Geometry: final body of the model. Coordinates: model frame, mm. Face numbers are marked on the shaded views. A direction names the side the tool comes from. Coordinates: 2 decimals unless noted, no trailing zeros. Order: outer loops, then holes, each group sorted by start corner. A loop starts at its lowest first (then second) coordinate and runs counter-clockwise, first axis right, second up. Notation, with made-up numbers: (79, -2) -> (127, -2) arc R19 ccw to (127, 18) -> close; hole circle Ø6 at (65, 46). An arc over 180 degrees is marked (long way). Use CSV: the item, a comma, the result in double quotes. Start each with the question number.
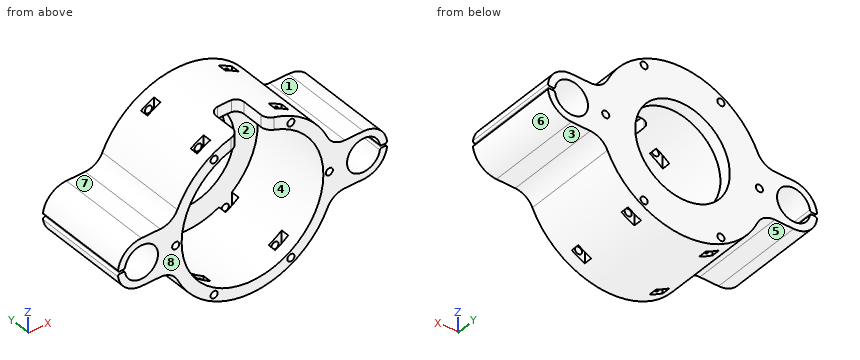
from build123d import *

# Parameters (mm, degrees)
F0_R           = 30
F1_DEPTH       = 35
F0_R_2         = 20
F2_DEPTH       = 5
F5_D           = 3
F4_W           = 12
F4_H           = 10.6380879879
F6_DEPTH       = 15
F7_R           = 3
F8_R           = 0.7
F9_R           = 0.8
F10_W          = 5.5
F10_H          = 3.5
F11_DEPTH      = 50
F11_DEPTH_BACK = 50


with BuildPart() as f1:
    # F0 (on Front) → F1 (new body)
    with BuildSketch(Plane.XZ):
        with BuildLine():
            ThreePointArc((-42.3231782953, 0.5), (-28.3410582734, 0), (-42.3231782953, -0.5))
            Line((-42.3231782953, -0.5), (-45.3285504511, -0.5))
            ThreePointArc((-45.3285504511, -0.5), (-42.2330826494, -7.2456883731), (-35.3410582734, -10))
            Line((-35.3410582734, -10), (-27.3923066529, -10))
            ThreePointArc((-27.3923066529, -10), (-23.0789957248, -11.2623929443), (-20.1269581172, -14.6511627907))
            ThreePointArc((-20.1269581172, -14.6511627907), (11.6589417266, -35), (43.4448415704, -14.6511627907))
            ThreePointArc((43.4448415704, -14.6511627907), (46.396879178, -11.2623929443), (50.7101901061, -10))
            Line((50.7101901061, -10), (58.6589417266, -10))
            ThreePointArc((58.6589417266, -10), (65.5509661026, -7.2456883731), (68.6464339043, -0.5))
            Line((68.6464339043, -0.5), (65.6410617485, -0.5))
            ThreePointArc((65.6410617485, -0.5), (51.6589417266, 0), (65.6410617485, 0.5))
            Line((65.6410617485, 0.5), (68.6464339043, 0.5))
            ThreePointArc((68.6464339043, 0.5), (65.5509661026, 7.2456883731), (58.6589417266, 10))
            Line((58.6589417266, 10), (50.7101901061, 10))
            ThreePointArc((50.7101901061, 10), (46.396879178, 11.2623929443), (43.4448415704, 14.6511627907))
            ThreePointArc((43.4448415704, 14.6511627907), (11.6589417266, 35), (-20.1269581172, 14.6511627907))
            ThreePointArc((-20.1269581172, 14.6511627907), (-23.0789957248, 11.2623929443), (-27.3923066529, 10))
            Line((-27.3923066529, 10), (-35.3410582734, 10))
            ThreePointArc((-35.3410582734, 10), (-42.2330826494, 7.2456883731), (-45.3285504511, 0.5))
            Line((-45.3285504511, 0.5), (-42.3231782953, 0.5))
        make_face()
        with Locations((11.6589417266, 0)):
            Circle(F0_R, mode=Mode.SUBTRACT)
    extrude(amount=F1_DEPTH)

    # F0 (on Front) → F2 (join)
    with BuildSketch(Plane.XZ):
        with BuildLine():
            ThreePointArc((-42.3231782953, 0.5), (-28.3410582734, 0), (-42.3231782953, -0.5))
            Line((-42.3231782953, -0.5), (-45.3285504511, -0.5))
            ThreePointArc((-45.3285504511, -0.5), (-42.2330826494, -7.2456883731), (-35.3410582734, -10))
            Line((-35.3410582734, -10), (-27.3923066529, -10))
            ThreePointArc((-27.3923066529, -10), (-23.0789957248, -11.2623929443), (-20.1269581172, -14.6511627907))
            ThreePointArc((-20.1269581172, -14.6511627907), (11.6589417266, -35), (43.4448415704, -14.6511627907))
            ThreePointArc((43.4448415704, -14.6511627907), (46.396879178, -11.2623929443), (50.7101901061, -10))
            Line((50.7101901061, -10), (58.6589417266, -10))
            ThreePointArc((58.6589417266, -10), (65.5509661026, -7.2456883731), (68.6464339043, -0.5))
            Line((68.6464339043, -0.5), (65.6410617485, -0.5))
            ThreePointArc((65.6410617485, -0.5), (51.6589417266, 0), (65.6410617485, 0.5))
            Line((65.6410617485, 0.5), (68.6464339043, 0.5))
            ThreePointArc((68.6464339043, 0.5), (65.5509661026, 7.2456883731), (58.6589417266, 10))
            Line((58.6589417266, 10), (50.7101901061, 10))
            ThreePointArc((50.7101901061, 10), (46.396879178, 11.2623929443), (43.4448415704, 14.6511627907))
            ThreePointArc((43.4448415704, 14.6511627907), (11.6589417266, 35), (-20.1269581172, 14.6511627907))
            ThreePointArc((-20.1269581172, 14.6511627907), (-23.0789957248, 11.2623929443), (-27.3923066529, 10))
            Line((-27.3923066529, 10), (-35.3410582734, 10))
            ThreePointArc((-35.3410582734, 10), (-42.2330826494, 7.2456883731), (-45.3285504511, 0.5))
            Line((-45.3285504511, 0.5), (-42.3231782953, 0.5))
        make_face()
        with Locations((11.6589417266, 0)):
            Circle(F0_R, mode=Mode.SUBTRACT)
        with Locations((11.6589417266, 0)):
            Circle(F0_R)
        with Locations((11.6589417266, 0)):
            Circle(F0_R_2, mode=Mode.SUBTRACT)
    extrude(amount=-F2_DEPTH)

    # F5 (through all)
    with Locations(Plane.XZ.offset(35)):
        with Locations((-4.5905371539, 28.1467282284), (27.910505085, 28.1467282284), (44.1610262045, 0), (27.910505085, -28.1467282284), (-4.5905371539, -28.1467282284), (-20.8410582734, 0)):
            Hole(F5_D / 2)

    # F4 (on offset) → F6 (cut)
    with BuildSketch(Plane.XZ.offset(35)):
        with Locations((11.6610262045, 32.1714654565)):
            Rectangle(F4_W, F4_H)
    extrude(amount=-F6_DEPTH, mode=Mode.SUBTRACT)

    # F7
    f7_edges = [f1.edges().sort_by_distance(p)[0] for p in [
        (5.661026, -20, 31.938272),
        (17.661026, -20, 31.937484),
        (5.661026, -35, 31.938272),
        (17.661026, -35, 31.937484),
    ]]
    fillet(f7_edges, radius=F7_R)

    # F8
    f8_edges = [f1.edges().sort_by_distance(p)[0] for p in [
        (68.646434, -15, 0.5),
        (68.646434, -15, -0.5),
        (65.641062, -15, -0.5),
        (65.641062, -15, 0.5),
    ]]
    fillet(f8_edges, radius=F8_R)

    # F9
    f9_edges = [f1.edges().sort_by_distance(p)[0] for p in [
        (-42.323178, -15, 0.5),
        (-42.323178, -15, -0.5),
        (-45.32855, -15, 0.5),
        (-45.32855, -15, -0.5),
    ]]
    fillet(f9_edges, radius=F9_R)

    # F10 (on Top) → F11 (cut, two sides)
    with BuildSketch(Plane.XY) as f11_sk:
        with Locations((-5, -28.25)):
            Rectangle(F10_W, F10_H)
        with Locations((28, -28.25)):
            Rectangle(F10_W, F10_H)
        with Locations((-5, -1.75)):
            Rectangle(F10_W, F10_H)
        with Locations((28, -1.75)):
            Rectangle(F10_W, F10_H)
    extrude(amount=F11_DEPTH, mode=Mode.SUBTRACT)
    extrude(f11_sk.sketch, amount=-F11_DEPTH_BACK, mode=Mode.SUBTRACT)


solid = f1.part
(1) Mould query, pull axis Z, two halves, no side actions, for the marked faces 1, 2 and 3. Classes: pulls with the +Z half, pulls with the -Z half, needs draft (parallel to the pull), parting line crosses it, or undercut.
(2) Section B-B (z = -3.5). Return loops of the section in (x, y), then the cut area to 3 significant figures.
(3) Section C-C (z = -17). Return loops of the section in (x, y), then the cut area to 3 significant figures.
(4) Section D-D (x = 35.5). Return loops of the section in (y, z), then the cut area to 3 significant figures.
(5) Access query for the marked faces 4, 5, 6, 7 and 8. Directions: +Z, -Z, +X, -X, +Y, -Y. A direction counts if a zero-diameter tool reaches every point of the face in a straight line with its end or side. Return the directions, or none.
(6) Section A-A (x = 61.5). Return loops of the section in (y, z), then the cut area to 3 significant figures.
(7) Line query: line 1 (X direction, y = -29, z = -2.5); line 2 (X direction, y = -4.5, z = 3); line 3 (Y direction, x = 35.5, z = -7.5). Output: solid intervals per line, ascending. Write a range as from..to.
(8) First-contact query: pin 1 (1.5 mm diameter, centred on x = -22, z = 16, fed in from -Y); pin 2 (5 mm diameter, centred on y = -6, z = -14.5, fed in from -X); pin 3 (6 mm diameter, centred on x = 5, y = -28, fed in from +Z); pin 4 (1 mm diameter, centred on y = -1.5, z = -27, fed in from +X). Flat tips, straight axial feed; report the tip coordinate or a pass-through.
Check sheet entries:
1,face 1,"pulls with the +Z half"
1,face 2,"undercut"
1,face 3,"pulls with the -Z half"
2,outline,"(-44.71, -35) -> (-41.4, -35) -> (-41.4, 5) -> (-44.71, 5) -> close; (-29.28, -35) -> (-18.14, -35) -> (-18.14, 0) -> (-8.03, 0) -> (-8.03, 5) -> (-29.28, 5) -> close; (31.35, 0) -> (41.45, 0) -> (41.45, -35) -> (52.6, -35) -> (52.6, 5) -> (31.35, 5) -> close; (64.72, -35) -> (68.03, -35) -> (68.03, 5) -> (64.72, 5) -> close"
2,area,"1,260 mm^2"
3,outline,"(-18.94, -35) -> (-13.06, -35) -> (-13.06, 0) -> (1.12, 0) -> (1.12, 5) -> (-18.94, 5) -> close; (22.19, 0) -> (36.38, 0) -> (36.38, -35) -> (42.25, -35) -> (42.25, 5) -> (22.19, 5) -> close"
3,area,"612 mm^2"
4,outline,"(-35, -25.62) -> (5, -25.62) -> (5, 25.62) -> (-35, 25.62) -> (-35, 18.21) -> (0, 18.21) -> (0, -18.21) -> (-35, -18.21) -> close"
4,area,"775 mm^2"
5,face 4,"-Y"
5,face 5,"-Z, -X, +Y, -Y"
5,face 6,"-Z, +X, +Y, -Y"
5,face 7,"+Z, -X, +Y, -Y"
5,face 8,"+Z, -Z, +X, -X, -Y"
6,outline,"(-35, -9.59) -> (5, -9.59) -> (5, -6.4) -> (-35, -6.4) -> close; (-35, 6.4) -> (5, 6.4) -> (5, 9.59) -> (-35, 9.59) -> close"
6,area,"255 mm^2"
7,line 1,"x = -45.02..-41.88, -28.8..-18.24, 41.55..52.12, 65.2..68.34"
7,line 2,"x = -44.88..-41.67, -29.02..-18.19, 41.51..52.33, 64.98..68.2"
7,line 3,"y = 0..5"
8,pin 1,"passes through"
8,pin 2,"stops at x = -22.1"
8,pin 3,"stops at z = 34.48"
8,pin 4,"stops at x = 34.52"
